Autodesk Inventor part; units mm, degrees
ref_plane "Work Plane1" through (0, 0, 0) normal (0, 1, 0) x (-1, 0, 0)
ref_plane "Work Plane2" through (0, 0, 12.5) normal (0, 0, 1) x (1, 0, 0)
ref_plane "YZ Plane" through (0, 0, 0) normal (1, 0, 0) x (0, 1, 0)
sketch "Sketch1" plane through (0, 0, 0) normal (0, 0, 1) x (1, 0, 0)
  line L0 (0, 0) -> (0, 13)
  line L1 (0, 13) -> (9, 13)
  line L2 (9, 13) -> (9, 8)
  line L3 (9, 8) -> (13, 8)
  line L4 (13, 8) -> (13, 0)
  line L5 (13, 0) -> (0, 0)
  dimension "d0" = 16
  dimension "d1" = 9
  dimension "d2" = 4
  dimension "d3" = 26
revolve "Revolution1" add sketch "Sketch1" angle 360 about axis through (13, 0, 0) along (-1, 0, 0)
sketch "Sketch2" plane through (0, 0, 0) normal (-1, 0, 0) x (0, 0, 1)
  line L0 (0, 0) -> (7.0711, 7.0711) construction
  line L1 (0, 0) -> (13, 0) construction
  circle A0 centre (0, 0) radius 13
  circle A1 centre (0, 0) radius 10 construction
  dimension "d6" = 20
  dimension "d5" = 45
hole "Hole1" at (0, 7.0711, 7.0711) direction (1, 0, 0) diameter 2 depth 9
pattern_circular "Circular Pattern1" count 4 over 360 about axis through (4.5, 0, 0) along (-1, 0, 0) of "Hole1"
sketch "Sketch3" plane through (0, 0, 0) normal (-1, 0, 0) x (0, 0, 1)
  circle A0 centre (0, 0) radius 13
  point P0 (0, 0)
hole "Hole2" at (0, 0, 0) direction (1, 0, 0) diameter 10 depth 13
chamfer "Chamfer1" distance 1 angle 45 1 edges at (0, -13, 0)
ref_plane "Work Plane1" through (0, 0, 0) normal (0, 1, 0) x (-1, 0, 0)
sketch "Sketch4" plane through (0, 0, 0) normal (0, 1, 0) x (-1, 0, 0)
  line L0 (-13, -5) -> (-13, 5)
  line L1 (-13, -8) -> (-13, 8)
  line L2 (-7, 7) -> (-4.8162, 13)
  line L3 (-9, 13) -> (-1, 13)
  line L4 (-13, 5) -> (0, 5)
  point P0 (0, 0)
  dimension "d28" = 20
  dimension "d29" = 2
  dimension "d34" = 2
ref_plane "Work Plane2" through (0, 0, 12.5) normal (0, 0, 1) x (1, 0, 0)
sketch "Sketch5" plane through (0, 0, 12.5) normal (0, 0, 1) x (1, 0, 0)
  circle A0 centre (4.8162, 0) radius 2
  point P0 (0, 0)
  dimension "d31" = 4
sweep "Sweep1" cut profiles "Sketch5" path "Sketch4" path curves L2
properties part number "08"
Model file for the job. Use its own axes, mm. A direction names the side the tool comes from. Give positions to 0.01 mm unless a question says otherwise; leave off trailing zeros. Write each loop counter-clockwise with the first axis right and the second up, starting at its lowest first coordinate (ties: lowest second). Pieces come first, ordered by that corner, then holes. Notation, with made-up numbers: M 60,-13 L 67,-13 A28 cw 67,17 Z; hole C 44.25,-14.75 d8. An arc over 180 degrees is marked long. Use a Markdown table: item, result.
1) Cut at B-B (x = 1.5). List the corners of the cut face in (y, z).
Responses:
| item | result |
|---|---|
| outline | C 0,0 d26; hole C -7.07,-7.07 d2; hole C -7.07,7.07 d2; hole C 0,0 d10; hole C 7.07,-7.07 d2; hole C 7.07,7.07 d2 |
2) Cut at C-C (x = 3.25). Give the number of separate pieces and of enclosed holes in the cut face, and give its area (3 significant figures).
Responses:
| item | result |
|---|---|
| separate pieces | 1 |
| enclosed holes | 5 |
| area | 437 mm2 |
3) Pin check, flat tips, straight feed: pin 1 (1.6 mm diameter, centred on y = -7.07, z = -7.07, fed in from -X); pin 2 (2.5 mm diameter, centred on y = 7.07, z = -7.07, fed in from +X); pin 3 (4 mm diameter, centred on x = 11.5, z = 7.5, fed in from -Y); pin 4 (6 mm diameter, centred on x = 2.5, z = 5, fed in from +Y). Stop position of each tip, or through.
Responses:
| item | result |
|---|---|
| pin 1 | passes through |
| pin 2 | stops at x = 9 |
| pin 3 | stops at y = -5.81 |
| pin 4 | stops at y = 12.85 |
4) Pull direction Y, two halves, no side cores. Call faces 1 (the cylindrical face through (11.03, -1.73, -7.81)), 2 (the flat face through (13, -0.1, 5.2)), 3 (the cylindrical face through (4.56, -6.08, -6.94)), 4 (the cylindrical face through (6.59, 4.88, -1.08)): +Y half, -Y half, draft (parallel to the pull), parting line (faces both ways), or undercut.
Responses:
| item | result |
|---|---|
| face 1 | parting line |
| face 2 | draft |
| face 3 | undercut |
| face 4 | undercut |
5) Cut at A-A (z = 0). List the corners of the cut face in (x, y), and give its area (3 significant figures).
Responses:
| item | result |
|---|---|
| outline | M 0,-12 L 1,-13 L 9,-13 L 9,-8 L 13,-8 L 13,-5 L 0,-5 Z; M 0,5 L 13,5 L 13,8 L 9,8 L 9,13 L 1,13 L 0,12 Z |
| area | 167 mm2 |
6) Drill centre lines: line 1 (Y direction, x = 5.5, z = 0); line 2 (Z direction, x = 10.25, y = 0); line 3 (X direction, y = 9, z = -5.5). Where is each one in solid material? Low to high. Write a range as from..to.
Responses:
| item | result |
|---|---|
| line 1 | y = -13..-5, 5..13 |
| line 2 | z = -8..-5, 5..8 |
| line 3 | x = 0..9 |
7) Tool access for faces 5 (the flat face through (9, 6, -6)), 6 (the flat face through (7, 0, 7)), 7 (the cylindrical face through (5.06, -2.82, -12.69)): list every direction of +Z, -Z, +X, -X, +Y, -Y with a clear straight run to the whole face (end or side of a thin tool).
Responses:
| item | result |
|---|---|
| face 5 | +X |
| face 6 | none |
| face 7 | +X, -X |
